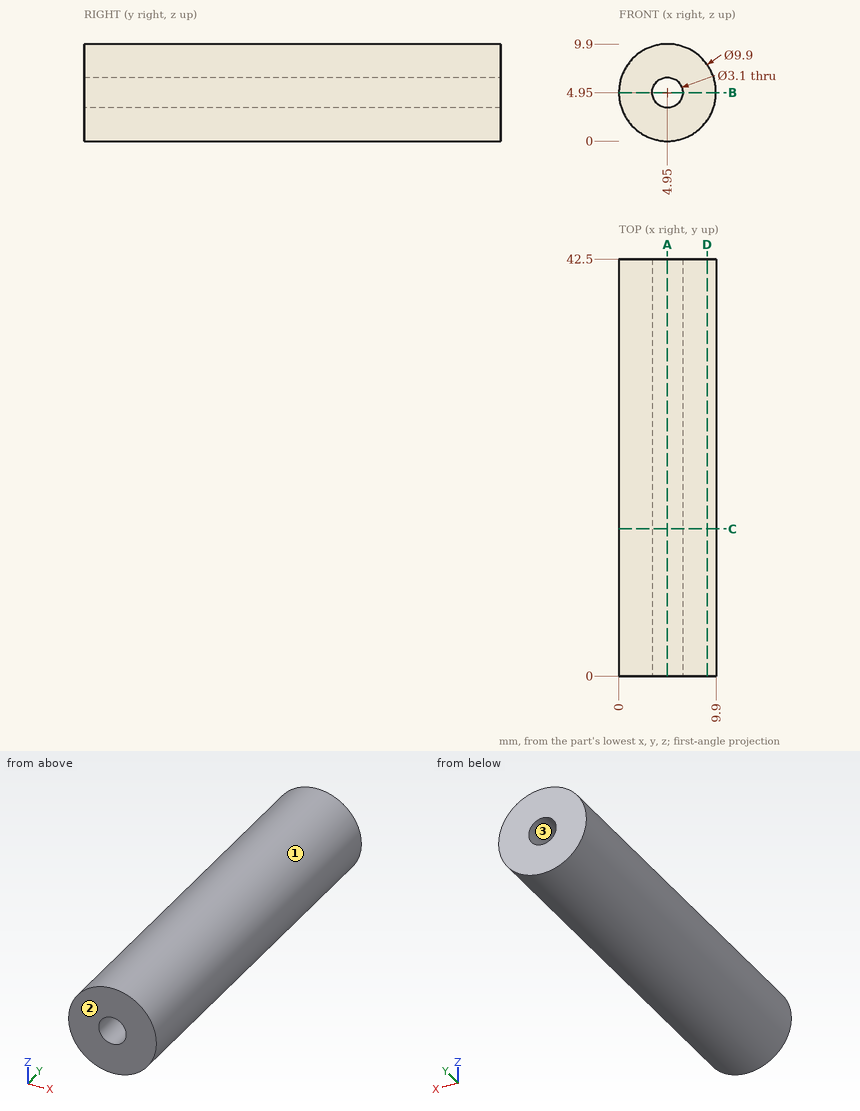
Input: dimensioned drawing with shaded views. Units: mm. Origin: part minimum x, y, z. Coordinates: 2 decimals unless noted, no trailing zeros. Order: outer loops, then holes, each group sorted by start corner. A loop starts at its lowest first (then second) coordinate and runs counter-clockwise, first axis right, second up. Notation, with made-up numbers: M 89,69.25 L 138,69.25 A29 ccw 138,104.25 Z; hole C 36.5,14 d10. An arc over 180 degrees is marked long. Answer as CSV lines item,"result".
Q1. Section B-B on z = 4.95. Return the cut outline in (x, y), and give its area (3 significant figures).
Answers:
outline,"M 0,0 L 3.4,0 L 3.4,42.5 L 0,42.5 Z; M 6.5,0 L 9.9,0 L 9.9,42.5 L 6.5,42.5 Z"
area,"289 mm^2"
Q2. Draft query along Z for the marked faces 1, 2 and 3. Return one class per face: pulls with the +Z half, pulls with the -Z half, needs draft (parallel to the pull), parting line crosses it, or undercut.
Answers:
face 1,"parting line crosses it"
face 2,"needs draft"
face 3,"undercut"
Q3. Section C-C on y = 15. Return the cut outline in (x, z), and give its area (3 significant figures).
Answers:
outline,"C 4.95,4.95 d9.9; hole C 4.95,4.95 d3.1"
area,"69.4 mm^2"
Q4. First-contact query: P1, Ø5, axis at y = 27.5, z = 3.5, coming from the -X side; P2, Ø1, axis at y = 13, z = 8, coming from the +X side. Flat tips, straight axial feed; report the tip coordinate or a pass-through.
Answers:
P1,"stops at x = 0"
P2,"stops at x = 9.19"
Q5. Section A-A on x = 4.95. Return the cut outline in (y, z).
Answers:
outline,"M 0,0 L 42.5,0 L 42.5,3.4 L 0,3.4 Z; M 0,6.5 L 42.5,6.5 L 42.5,9.9 L 0,9.9 Z"
Q6. Line query: probe 1 along X at (y, z) = (19.5, 4.95); probe 2 along Z at (x, y) = (6, 4); probe 3 along X at (y, z) = (12, 4.5). Output: solid intervals per line, ascending. Write a range as [from, to].
Answers:
probe 1,"x = [0, 3.4], [6.5, 9.9]"
probe 2,"z = [0.11, 3.81], [6.09, 9.79]"
probe 3,"x = [0.02, 3.47], [6.43, 9.88]"
Q7. Section D-D on x = 9. Return the cut outline in (y, z), and give its area (3 significant figures).
Answers:
outline,"M 0,2.1 L 42.5,2.1 L 42.5,7.8 L 0,7.8 Z"
area,"242 mm^2"
